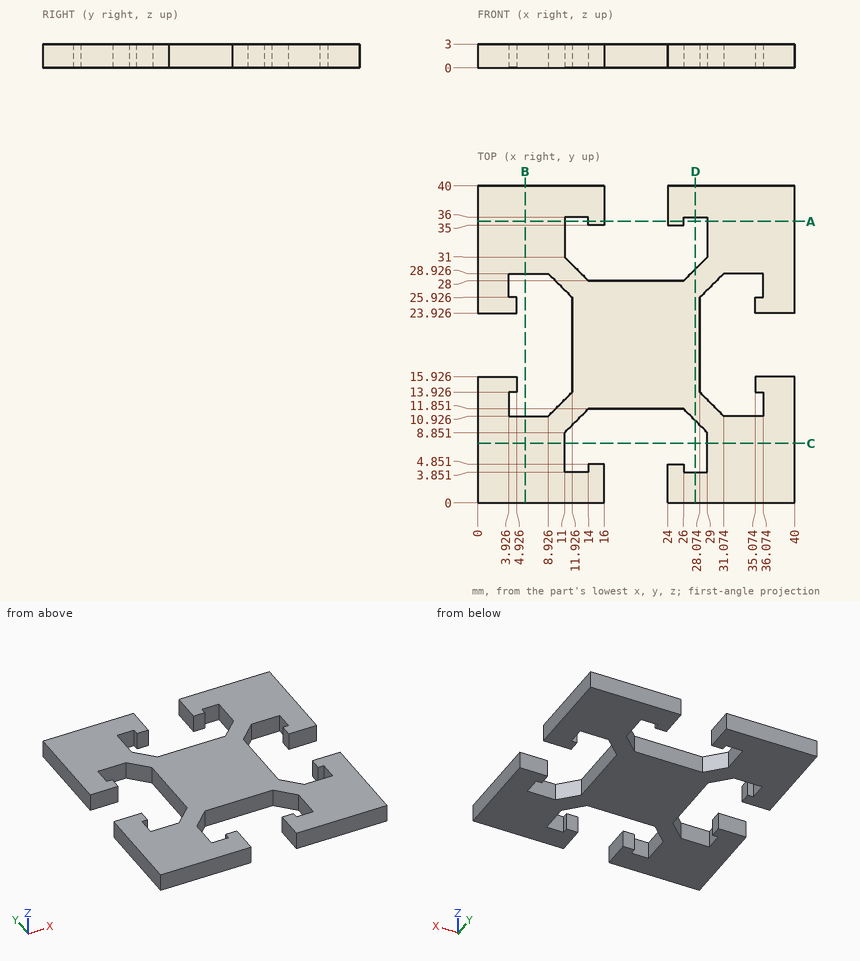
The drawing under review shows one solid part. Ordinate dimensions are in mm from its lowest x, y, z. Round coordinates to 2 decimals unless told otherwise and drop trailing zeros. Loops run counter-clockwise (first coordinate to the right, second up) from the corner with the lowest first, then second, coordinate; pieces in that order, holes last. Notation, with made-up numbers: (31.25, 64.25) - (78.25, 64.25) arc R25 ccw to (78.25, 78.25) - close; hole circle Ø9 at (37, 58.25). An arc over 180 degrees is marked (long way). Use a Markdown table: item, result. Add a question column.
Q1. For probe 1 along Y at (x, z) = (36, 1.9) (1 decimal); probe 2 along X at (y, z) = (14, 2.6) (1 decimal); probe 3 along X at (y, z) = (7, 1.7), list the stretches that pass through material, from the lowest coordinate up.
Q2. Add section B-B (x = 6). State the section outline as (y, z) points (1 decimal), plus the area to 3 significant figures.
Q3. Add section C-C (y = 7.5). State the section outline as (x, z) points, plus the area to 3 significant figures.
Q4. Insertion check: pin 1 Ø0.9 at (x, z) = (21, 1) entering from +Y. The pin has a flat end and moves straight along its axis. Give the tip position at first contact, or say it passes through.
Q5. Add section A-A (y = 35.5). State the section outline as (x, z) points.
Q6. Add section D-D (x = 27.5). State the section outline as (y, z) points.
Worked answers:
| question | item | result |
|---|---|---|
| 1 | probe 1 | 0 to 10.9, 13.9 to 15.9, 23.9 to 25.9, 28.9 to 40 |
| 1 | probe 2 | 0 to 4.9, 11.9 to 28.1, 35.1 to 40 |
| 1 | probe 3 | 0 to 11, 29 to 40 |
| 2 | outline | (0, 0) - (10.9, 0) - (10.9, 3) - (0, 3) - close; (28.9, 0) - (40, 0) - (40, 3) - (28.9, 3) - close |
| 2 | area | 66.0 mm² |
| 3 | outline | (0, 0) - (11, 0) - (11, 3) - (0, 3) - close; (29, 0) - (40, 0) - (40, 3) - (29, 3) - close |
| 3 | area | 66.0 mm² |
| 4 | pin 1 | y = 28 |
| 5 | outline | (0, 0) - (11, 0) - (11, 3) - (0, 3) - close; (14, 0) - (16, 0) - (16, 3) - (14, 3) - close; (24, 0) - (26, 0) - (26, 3) - (24, 3) - close; (29, 0) - (40, 0) - (40, 3) - (29, 3) - close |
| 6 | outline | (0, 0) - (3.85, 0) - (3.85, 3) - (0, 3) - close; (10.35, 0) - (29.5, 0) - (29.5, 3) - (10.35, 3) - close; (36, 0) - (40, 0) - (40, 3) - (36, 3) - close |
